CAD build for the part. Positions are in the model's coordinates, mm. A direction names the side the tool comes from. Give positions to 0.01 mm unless a question says otherwise; leave off trailing zeros. Loops run counter-clockwise (first coordinate to the right, second up) from the corner with the lowest first, then second, coordinate; pieces in that order, holes last. Notation, with made-up numbers: M 38,49.25 L 78,49.25 A16 ccw 78,79.25 Z; hole C 85,51.5 d5. An arc over 180 degrees is marked long. Answer as CSV lines item,"result".
Autodesk Fusion 360 part; units mm, degrees
sketch "Esquisse1" plane through (0, 0, 0) normal (0, 0, 1) x (1, 0, 0)
  circle A0 centre (16.25, 10) radius 1.65
  circle A1 centre (16.25, 61) radius 1.65
  circle A2 centre (67.25, 10) radius 1.95
  circle A3 centre (67.25, 61) radius 1.95
  line L0 (67.25, 61) -> (16.25, 10) construction
  line L1 (16.25, 61) -> (67.25, 10) construction
  circle A4 centre (41.75, 35.5) radius 30.5 construction
  circle A5 centre (16.25, 61) radius 5
  circle A6 centre (16.25, 10) radius 5
  arc A7 (19.7855, 57.4645) -> (19.7855, 13.5355) centre (41.75, 35.5) ccw
  line L2 (16.5063, 65.9934) -> (0, 65.9934)
  line L3 (0, 65.9934) -> (0, 0)
  line L4 (0, 0) -> (7.5, 0)
  line L5 (16.25, 10) -> (16.25, 5)
  line L6 (16.25, 5) -> (7.5, 0)
  line L7 (7.5, 0) -> (7.5, 15)
  line L8 (7.5, 15) -> (0, 15)
  dimension "d1" = 3.3
  dimension "d2" = 3.3
  dimension "d3" = 16.25
  dimension "d4" = 16.25
  dimension "d5" = 51
  dimension "d6" = 10
  dimension "d7" = 3.9
  dimension "d8" = 51
  dimension "d9" = 3.9
  dimension "d10" = 51
  dimension "d11" = 51
  dimension "d12" = 61
  dimension "d13" = 10
  dimension "d14" = 10
  dimension "d15" = 7.5
  dimension "d16" = 15
extrude "Extrusion1" add sketch "Esquisse1" along normal blind 22 contours L3 L4 L7 L8 makes body 1
extrude "Extrusion2" add sketch "Esquisse1" along normal blind 5 separate body contours A6 | A5 A6 A7 L2 L3 L6 L7 L8 | A5 L2 picked at (18.7618, 58.051) makes body 2
sketch "Esquisse2" plane through (0, 0, 0) normal (-1, 0, 0) x (0, -1, 0)
  line L0 (-15, 0) -> (0, 0)
  line L1 (0, 0) -> (0, 22)
  line L2 (0, 22) -> (-15, 22)
  line L3 (-15, 22) -> (-15, 0)
  circle A0 centre (-7.5, 14.5) radius 2.5
  arc A1 (0, 14.5) -> (-7.5, 22) centre (-7.5, 14.5) ccw
  arc A2 (-7.5, 22) -> (-15, 14.5) centre (-7.5, 14.5) ccw
  dimension "d21" = 5
  dimension "d22" = 7.5
  dimension "d23" = 7.5
extrude "Extrusion3" cut sketch "Esquisse2" against normal blind 8 contours L2 L3 A2 | L1 L2 A1 | A0 bodies 1
sketch "Esquisse3" plane through (0, 0, 5) normal (0, 0, 1) x (-1, 0, 0)
  circle A0 centre (-16.25, -61) radius 1.65
  circle A1 centre (-16.25, -10) radius 1.65
  arc A2 (-16.25, -5) -> (-19.7855, -13.5355) centre (-16.25, -10) ccw
  arc A3 (-19.7855, -57.4645) -> (-19.7855, -13.5355) centre (-41.75, -35.5) ccw
  arc A4 (-19.7855, -57.4645) -> (-16.5063, -65.9934) centre (-16.25, -61) ccw
  line L0 (-16.5063, -65.9934) -> (0, -65.9934)
  line L1 (0, -65.9934) -> (0, -15)
  line L2 (0, -15) -> (-7.5, -15)
  line L3 (-7.5, -15) -> (-7.5, 0)
  line L4 (-7.5, 0) -> (-16.25, -5)
  line L5 (0, -35.5) -> (-5, -66.0689)
  line L6 (-5, -66.0689) -> (0, -65.9934)
  line L7 (0, -35.5) -> (0, -65.9934)
  dimension "d27" = 5
extrude "Extrusion4" cut sketch "Esquisse3" against normal blind 10 contours L0 L1 L5 L7 bodies 2
mirror "Symétrie miroir2" about plane through (0, 65.9934, 0) normal (-1, 0, 0) of bodies 2 1 merged
sketch "Esquisse4" plane through (0, 0, 0) normal (0, 0, 1) x (1, 0, 0)
  line L0 (0, 0) -> (31.9819, 0)
  line L1 (31.9819, 0) -> (31.9819, 68.443)
  line L2 (31.9819, 68.443) -> (0, 68.443)
  line L3 (0, 68.443) -> (0, 0)
extrude "Extrusion5" cut sketch "Esquisse4" sketch "Esquisse1" along normal blind 30 of sketch 2 contours A5 A6 A7 L2 L3 L6 L7 L8 | L3 L4 L7 L8 | A5 L2 picked at (18.7618, 58.051) bodies 1 2
combine "Combiner1" operation add target body 1 tool bodies 2
equation "d3 = 14.3 mm + 1.95 mm"
Q1. Pin check, flat tips, straight feed: P1, Ø5, axis at y = 18, z = 4.5, coming from the -X side; P2, Ø12, axis at y = 8, z = 16, coming from the -X side; P3, Ø10, axis at x = -3.5, y = 49.5, coming from the -Z side; P4, Ø6, axis at x = -3, z = 9, coming from the +Y side. Stop position of each tip, or through.
Solution:
P1,"stops at x = -17.98"
P2,"stops at x = -7.5"
P3,"stops at z = 0"
P4,"stops at y = 15"
Q2. Cut at A-A (y = 61). Write the cut outline in (x, z).
Solution:
outline,"M -21.25,0 L -17.9,0 L -17.9,5 L -21.25,5 Z; M -14.6,0 L -4.17,0 L -4.17,5 L -14.6,5 Z"
Q3. Cut at B-B (z = 1.5). Write the cut outline in (x, y), and give its area (3 significant figures).
Solution:
outline,"M -19.79,13.54 A5 ccw -16.25,5 L -7.5,0 L 0,0 L 0,35.5 L -4.99,65.99 L -16.51,65.99 A5 ccw -19.79,57.46 A31.06 cw Z; hole C -16.25,10 d3.3; hole C -16.25,61 d3.3"
area,"909 mm²"
Q4. Cut at D-D (x = -13). Write the cut outline in (y, z).
Solution:
outline,"M 3.14,0 L 23.74,0 L 23.74,5 L 3.14,5 Z; M 47.26,0 L 65.99,0 L 65.99,5 L 47.26,5 Z"
Q5. Mould opens along Y. For faces 4 (the flat face through (-11.814, 2.465, 2.465)), 5 (the flat face through (-2.53, 50.96, 2.54)), 6 (the cylindrical face through (-10.69, 35.84, 2.46)) say: released by +Y, released by -Y, zero draft, split by the parting line, or undercut.
Solution:
face 4,"released by -Y"
face 5,"released by +Y"
face 6,"undercut"
Q6. Cut at C-C (x = -1.25). Write the cut outline in (y, z), and give its area (3 significant figures).
Solution:
outline,"M 0,0 L 43.14,0 L 43.14,5 L 15,5 L 15,14.5 A7.5 ccw 0,14.5 Z; hole C 7.5,14.5 d5"
area,"427 mm²"
Q7. Which spindle directions (+Z, -Z, +X, -X, +Y, -Y) get a long thin tool onto all of the face, cutting with end or side? Do faces 1 (the flat face through (-4, 15, 10)), 2 (the flat face through (-7.5, 8, 11)), 3 (the cylindrical face through (-17.011, 59.536, 2.465)). Say none if no direction does.
Solution:
face 1,"+Z, +X, -X, +Y"
face 2,"+Z, -X, +Y, -Y"
face 3,"+Z, -Z"
Q8. Wall check: line 1 (X direction, y = 10, z = 2.75); line 2 (Z direction, x = -5.25, y = 7.5); line 3 (Y direction, x = -16.25, z = 2.1). Give the ranges that are in metal, low to high. Write a range as [from, to].
Solution:
line 1,"x = [-21.25, -17.9], [-14.6, 0]"
line 2,"z = [0, 12], [17, 22]"
line 3,"y = [5, 8.35], [11.65, 17.76], [53.24, 59.35], [62.65, 65.99]"
